Part model, mm, in its own coordinate system. A direction names the side the tool comes from. Round coordinates to 2 decimals unless told otherwise and drop trailing zeros. Order: outer loops, then holes, each group sorted by start corner. A loop starts at its lowest first (then second) coordinate and runs counter-clockwise, first axis right, second up. Notation, with made-up numbers: (51.5, -15.5) - (86.5, -15.5) arc R22 cw to (86.5, -1.5) - close; hole circle Ø6 at (36.5, 37.5). An arc over 180 degrees is marked (long way). Answer as a JSON object with one key per item and string values.
```python
from build123d import *

# Parameters (mm, degrees)
F0_W     = 25.4
F0_H     = 3.175
F1_DEPTH = 3.175
F2_W     = 3.175
F2_H     = 25.4
F3_DEPTH = 3.175
F4_W     = 1.778
F4_H     = 25.4
F4_H_2   = 28.575
F5_DEPTH = 3.175


with BuildPart() as f1:
    # F0 (on Front) → F1 (new body)
    with BuildSketch(Plane.XZ):
        Polygon((25.4, -39.8197), (50.8, -39.8197), (50.8, 61.7803), (-50.8, 61.7803), (-50.8, -39.8197), (-25.4, -39.8197), (0, -39.8197), align=None)
        with Locations((-12.7, -41.4072)):
            Rectangle(F0_W, F0_H)
        with Locations((38.1, -41.4072)):
            Rectangle(F0_W, F0_H)
    extrude(amount=F1_DEPTH)

    # F2 (on face) → F3 (join)
    with BuildSketch(Plane.XZ.offset(3.175)):
        with Locations((-52.3875, 23.6803)):
            Rectangle(F2_W, F2_H)
        with Locations((-52.3875, -27.1197)):
            Rectangle(F2_W, F2_H)
        with Locations((52.3875, 49.0803)):
            Rectangle(F2_W, F2_H)
        with Locations((52.3875, -1.7197)):
            Rectangle(F2_W, F2_H)
    extrude(amount=-F3_DEPTH)

    # F4 (on face) → F5 (cut)
    with BuildSketch(Plane(origin=(0, 0, 0), x_dir=(-1, 0, 0), z_dir=(0, 1, 0))):
        with Locations((-49.911, 23.6803)):
            Rectangle(F4_W, F4_H)
        with Locations((49.911, 49.0803)):
            Rectangle(F4_W, F4_H)
        with Locations((49.911, -1.7197)):
            Rectangle(F4_W, F4_H)
        with Locations((-49.911, -28.7072)):
            Rectangle(F4_W, F4_H_2)
    extrude(amount=-F5_DEPTH, mode=Mode.SUBTRACT)


solid = f1.part
```
Item 1: Cut at A-A (y = -0.5). Write the cut outline in (x, z) (3 decimals).
Taken from the geometry:
{"outline": "(-53.975, -39.82) - (-25.4, -39.82) - (-25.4, -42.995) - (0, -42.995) - (0, -39.82) - (25.4, -39.82) - (25.4, -42.995) - (49.022, -42.995) - (49.022, -14.42) - (53.975, -14.42) - (53.975, 10.98) - (49.022, 10.98) - (49.022, 36.38) - (53.975, 36.38) - (53.975, 61.78) - (-49.022, 61.78) - (-49.022, 36.38) - (-53.975, 36.38) - (-53.975, 10.98) - (-49.022, 10.98) - (-49.022, -14.42) - (-53.975, -14.42) - close"}
Item 2: Tool access for faces 1 (the flat face through (49.022, -2, -29)), 2 (the flat face through (-51, -2, 10.98)), 3 (the flat face through (52, -2, 10.98)): list every direction of +Z, -Z, +X, -X, +Y, -Y with a clear straight run to the whole face (end or side of a thin tool).
Taken from the geometry:
{"face 1": "-Z, +X, +Y, -Y", "face 2": "-X, +Y, -Y", "face 3": "+X, +Y, -Y"}
Item 3: Drop flat-ended pins along their axis: P1, Ø1.6, axis at x = -37, y = -1.5, coming from the -Z side; P2, Ø1.6, axis at y = -2, z = -26.5, coming from the +X side; P3, Ø1, axis at y = -2, z = -40.5, coming from the -X side; P4, Ø10, axis at x = -42, z = 31.5, coming from the +Y side. Give the stop position or say it passes through.
Taken from the geometry:
{"P1": "z = -39.82", "P2": "x = 49.02", "P3": "x = -25.4", "P4": "y = 0"}
Item 4: Two-plate mould, pull along X, no slides. Class faces 4 (the flat face through (51, -2, -14.42)), 5 (the flat face through (-53.975, -2, 24)), 6 (the flat face through (13, -2, -39.82)): pulls with the +X half, pulls with the -X half, needs draft (parallel to the pull), parting line crosses it, or undercut.
Taken from the geometry:
{"face 4": "needs draft", "face 5": "pulls with the -X half", "face 6": "undercut"}
Item 5: Cut at C-C (x = -28). Write the cut outline in (y, z) (3 decimals).
Taken from the geometry:
{"outline": "(-3.175, -39.82) - (0, -39.82) - (0, 61.78) - (-3.175, 61.78) - close"}
Item 6: Cut at B-B (z = -2.5). Write the cut outline in (x, y) (3 decimals).
Taken from the geometry:
{"outline": "(-49.022, -3.175) - (53.975, -3.175) - (53.975, 0) - (-49.022, 0) - close"}
Item 7: Probe L1, parallel to Z at x = -40.5, y = -1.9; L2, parallel to X at y = -0.75, z = -28 (3 decimals); L3, parallel to X at y = -2.7, z = 57 (3 decimals). List the from-to ranges inside material, lowest first. Write a range as from..to.
Taken from the geometry:
{"L1": "-39.82..61.78", "L2": "-53.975..49.022", "L3": "-49.022..53.975"}
